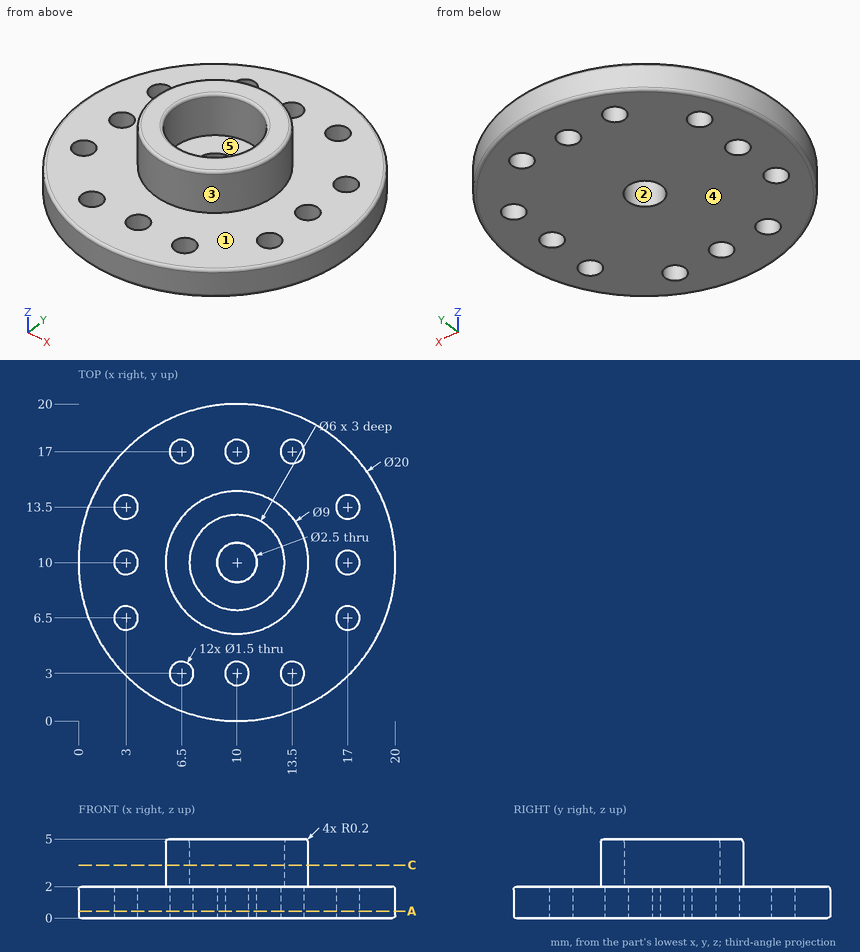
Print and shaded views of the part. All mm, measured from the part's lowest x, y and z. A direction names the side the tool comes from. Give positions to 0.01 mm unless a question says otherwise; leave off trailing zeros. Loops run counter-clockwise (first coordinate to the right, second up) from the corner with the lowest first, then second, coordinate; pieces in that order, holes last. Notation, with made-up numbers: (39.25, -33) - (44.25, -33) arc R14 cw to (44.25, -19) - close; hole circle Ø3 at (25.25, 56.5). An arc over 180 degrees is marked (long way). One line per item, written item: value. Start each with the question number.
1. Slice it at C-C (z = 3.35). List the corners of the cut face in (x, y), plus the area to 3 significant figures.
2. Pin check, flat tips, straight feed: pin 1 (3 mm diameter, centred on x = 10, y = 10, fed in from +Z); pin 2 (2 mm diameter, centred on y = 3.5, z = 2.5, fed in from -X); pin 3 (2 mm diameter, centred on x = 5, z = 2, fed in from +Y). Stop position of each tip, or through.
3. Pull direction Y, two halves, no side cores. Call the marked faces 1, 2 and 3: pulls with the +Y half, pulls with the -Y half, needs draft (parallel to the pull), parting line crosses it, or undercut.
4. Slice it at A-A (z = 0.45). Give the number of separate pieces and of enclosed holes in the cut face, plus the area to 3 significant figures.
5. Probe L1, parallel to Y at x = 10, z = 0.8; L2, parallel to Y at x = 10.5, z = 1; L3, parallel to Y at x = 13.5, z = 0.9. List the from-to ranges inside material, lowest first. Write a range as from..to.
6. Which spindle directions (+Z, -Z, +X, -X, +Y, -Y) get a long thin tool onto all of the face, cutting with end or side? Do the marked faces 4 and 5. Say none if no direction does.
Solution:
1. outline: circle Ø9 at (10, 10); hole circle Ø6 at (10, 10)
1. area: 35.3 mm^2
2. pin 1: stops at z = 2
2. pin 2: stops at x = 1.81
2. pin 3: stops at y = 19.16
3. face 1: needs draft
3. face 2: undercut
3. face 3: parting line crosses it
4. separate pieces: 1
4. enclosed holes: 13
4. area: 288 mm^2
5. L1: y = 0..2.25, 3.75..8.75, 11.25..16.25, 17.75..20
5. L2: y = 0.01..2.44, 3.56..8.85, 11.15..16.44, 17.56..19.99
5. L3: y = 0.63..2.25, 3.75..16.25, 17.75..19.37
6. face 4: -Z, +X, -X, +Y, -Y
6. face 5: +Z
